from build123d import *

# Parameters (mm, degrees)
BOSS_EXTRUDE1_DEPTH = 15.24
SKETCH5_R           = 3.5
CUT_EXTRUDE1_DEPTH  = 15.24
SKETCH6_R           = 1.778
CUT_EXTRUDE2_DEPTH  = 15.24
SKETCH8_W           = 3.175
SKETCH8_H           = 50.8
BOSS_EXTRUDE2_DEPTH = 6.35
SKETCH7_R           = 1.5
CUT_EXTRUDE3_DEPTH  = 6.35
CIRPATTERN1_COUNT   = 4
FILLET1_R           = 2.54


with BuildPart() as part:
    # Sketch2 → Boss-Extrude1 (new body)
    with BuildSketch(Plane.XY):
        Polygon((-27.94, 0), (27.94, 0), (27.94, 6.35), (-2.54, 6.35), (-2.54, 50.8), (-8.89, 50.8), (-8.89, 6.35), (-27.94, 6.35), align=None)
    extrude(amount=BOSS_EXTRUDE1_DEPTH)

    # Sketch5 → Cut-Extrude1 (cut)
    with BuildSketch(Plane.ZY.offset(8.89)):
        with Locations((7.62, 27.686)):
            Circle(SKETCH5_R)
    extrude(amount=-CUT_EXTRUDE1_DEPTH, mode=Mode.SUBTRACT)

    # Sketch6 → Cut-Extrude2 (cut)
    with BuildSketch(Plane(origin=(0, 6.35, 0), x_dir=(1, 0, 0), z_dir=(0, 1, 0))):
        with Locations((-25.146, -7.62)):
            Circle(SKETCH6_R)
        with Locations((-15.24, -7.62)):
            Circle(SKETCH6_R)
    extrude(amount=-CUT_EXTRUDE2_DEPTH, mode=Mode.SUBTRACT)

    # Sketch8 → Boss-Extrude2 (add)
    with BuildSketch(Plane.ZY.offset(8.89)):
        with Locations((-1.5875, 25.4)):
            Rectangle(SKETCH8_W, SKETCH8_H)
        with Locations((16.8275, 25.4)):
            Rectangle(SKETCH8_W, SKETCH8_H)
    extrude(amount=-BOSS_EXTRUDE2_DEPTH)

    # Sketch7 → Cut-Extrude3 (cut)
    with BuildSketch(Plane.ZY.offset(8.89)):
        with Locations((7.62, 34.186)):
            Circle(SKETCH7_R)
    cut_extrude3 = extrude(amount=-CUT_EXTRUDE3_DEPTH, mode=Mode.SUBTRACT)

    # CirPattern1: Cut-Extrude3 ×4 about axis
    cirpattern1_axis = Axis((0, 27.686, 7.62), (1, 0, 0))
    for i in range(1, CIRPATTERN1_COUNT):
        add(cut_extrude3.rotate(cirpattern1_axis, i * 360 / CIRPATTERN1_COUNT), mode=Mode.SUBTRACT)

    # Fillet1
    fillet1_edges = [part.edges().sort_by_distance(p)[0] for p in [
        (27.94, 3.175, 0),
        (-27.94, 3.175, 0),
        (27.94, 3.175, 15.24),
        (-5.715, 50.8, -3.175),
        (-27.94, 3.175, 15.24),
        (-5.715, 50.8, 18.415),
    ]]
    fillet(fillet1_edges, radius=FILLET1_R)


solid = part.part
CAD build for the part. Positions are in the model's coordinates, mm. A direction names the side the tool comes from. Round coordinates to 2 decimals unless told otherwise and drop trailing zeros. Order: outer loops, then holes, each group sorted by start corner. A loop starts at its lowest first (then second) coordinate and runs counter-clockwise, first axis right, second up. Notation, with made-up numbers: (25.5, 8.25) - (44.5, 8.25) arc R32 cw to (44.5, 43.25) - close; hole circle Ø8 at (-26.75, -1). An arc over 180 degrees is marked (long way). Return JSON: item names as keys, results as strings.
(1) Pull direction Y, two halves, no side cores. Call faces 5 (the face through (-5.759, 35.673, 7.425)), 6 (the face through (-5.759, 26.58, 0.106)), 7 (the face through (0, 0, 7)), 8 (the face through (-17, 3, 0)): +Y half, -Y half, draft (parallel to the pull), parting line (faces both ways), or undercut.
Answer key:
{"face 5": "undercut", "face 6": "undercut", "face 7": "-Y half", "face 8": "draft"}
(2) Cut at A-A (x = -15.24). Give the cut face in (y, z).
Answer key:
{"outline": "(0, 0) - (6.35, 0) - (6.35, 5.84) - (0, 5.84) - close; (0, 9.4) - (6.35, 9.4) - (6.35, 15.24) - (0, 15.24) - close"}
(3) Tool access for faces 1 (the face through (13, 6.35, 8)), 2 (the face through (-18, 6.35, 8)), 3 (the face through (-5.671, 50.076, 17.651)), 4 (the face through (11, 3, 0)): list every direction of +Z, -Z, +X, -X, +Y, -Y with a clear straight run to the whole face (end or side of a thin tool).
Answer key:
{"face 1": "+Z, -Z, +X, +Y", "face 2": "+Z, -Z, -X, +Y", "face 3": "+Z, +X, -X, +Y", "face 4": "-Z, +X, +Y, -Y"}
(4) Wall check: probe 1 along X at (y, z) = (3.25, 7.62); probe 2 along Z at (x, y) = (-15, 2); probe 3 along X at (y, z) = (11, 9.25). Give the ranges that are in metal, low to high. Write a range as from..to.
Answer key:
{"probe 1": "x = -27.94..-26.92, -23.37..-17.02, -13.46..27.94", "probe 2": "z = 0..5.86, 9.38..15.24", "probe 3": "x = -8.89..-2.54"}
(5) Cut at D-D (y = 28.5). Give the cut face in (x, z) (3 decimals).
Answer key:
{"outline": "(-8.89, -3.175) - (-2.54, -3.175) - (-2.54, -0.14) - (-8.89, -0.14) - close; (-8.89, 2.38) - (-2.54, 2.38) - (-2.54, 4.216) - (-8.89, 4.216) - close; (-8.89, 11.024) - (-2.54, 11.024) - (-2.54, 12.86) - (-8.89, 12.86) - close; (-8.89, 15.38) - (-2.54, 15.38) - (-2.54, 18.415) - (-8.89, 18.415) - close"}
(6) Pin check, flat tips, straight feed: pin 1 Ø3 at (x, y) = (17.5, 3.5) entering from -Z; pin 2 Ø1.5 at (y, z) = (38, 7) entering from +X; pin 3 Ø3 at (y, z) = (16, 11.5) entering from -X; pin 4 Ø1.5 at (x, z) = (12, 14.5) entering from -Y. Stop position of each tip, or through.
Answer key:
{"pin 1": "stops at z = 0", "pin 2": "stops at x = -2.54", "pin 3": "stops at x = -8.89", "pin 4": "stops at y = 0"}
(7) Cut at B-B (z = 7.62). Give the cut face in (x, y).
Answer key:
{"outline": "(-27.94, 0) - (-26.92, 0) - (-26.92, 6.35) - (-27.94, 6.35) - close; (-23.37, 0) - (-17.02, 0) - (-17.02, 6.35) - (-23.37, 6.35) - close; (-13.46, 0) - (27.94, 0) - (27.94, 6.35) - (-2.54, 6.35) - (-2.54, 19.69) - (-8.89, 19.69) - (-8.89, 6.35) - (-13.46, 6.35) - close; (-8.89, 22.69) - (-2.54, 22.69) - (-2.54, 24.19) - (-8.89, 24.19) - close; (-8.89, 31.19) - (-2.54, 31.19) - (-2.54, 32.69) - (-8.89, 32.69) - close; (-8.89, 35.69) - (-2.54, 35.69) - (-2.54, 50.8) - (-8.89, 50.8) - close"}
(8) Cut at C-C (y = 35). Give the cut face in (x, z) (3 decimals).
Answer key:
{"outline": "(-8.89, -3.175) - (-2.54, -3.175) - (-2.54, 6.36) - (-8.89, 6.36) - close; (-8.89, 8.88) - (-2.54, 8.88) - (-2.54, 18.415) - (-8.89, 18.415) - close"}
